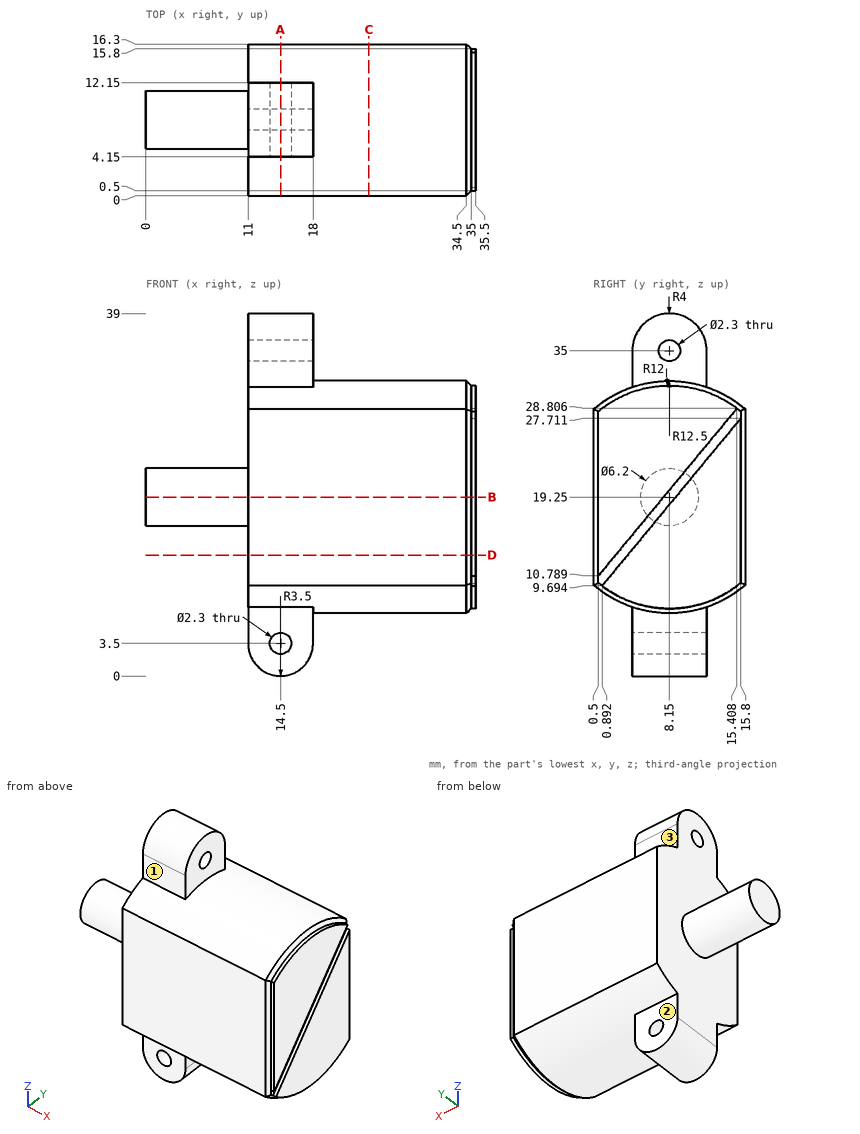
Source: three-view drawing plus pictorial views. Frame: mm from the lowest corner of the part. A direction names the side the tool comes from. Coordinates: 2 decimals unless noted, no trailing zeros. Order: outer loops, then holes, each group sorted by start corner. A loop starts at its lowest first (then second) coordinate and runs counter-clockwise, first axis right, second up.
Item 1: Set-up query: the marked faces 1, 2 and 3. Return all of +Z, -Z, +X, -X, +Y, -Y with unobstructed straight access to the full face (end or side cutting, diameter ignored); none if empty.
Output values:
face 1: +Z, +X, -X, -Y
face 2: -Z, +X, -X, +Y
face 3: +Z, +X, -X, +Y
Item 2: First-contact query: P1, Ø2, axis at y = 8.5, z = 4.5, coming from the +X side; P2, Ø8, axis at x = 27, y = 6.5, coming from the -Z side; P3, Ø2, axis at x = 8.5, z = 15.5, coming from the +Y side. Flat tips, straight axial feed; report the tip coordinate or a pass-through.
Output values:
P1: stops at x = 18
P2: stops at z = 6.75
P3: stops at y = 9.58
Item 3: Material intervals for line 1 (Y direction, x = 15, z = 35); line 2 (X direction, y = 8.5, z = 3.5); line 3 (Z direction, x = 14.5, y = 7.5), sorted ascending.
Output values:
line 1: y = 4.15 to 7, 9.3 to 12.15
line 2: x = 11 to 13.35, 15.65 to 18
line 3: z = 0 to 2.35, 4.65 to 34.05, 35.95 to 38.95
Item 4: Cut plane D-D (z = 13). Return loops of the section in (x, y).
Output values:
outline: (11, 0) - (34.5, 0) - (35, 0.5) - (35.5, 0.5) - (35.5, 2.33) - (35, 2.33) - (35, 3.63) - (35.5, 3.63) - (35.5, 15.8) - (35, 15.8) - (34.5, 16.3) - (11, 16.3) - close
Item 5: Cut plane A-A (x = 14.5). Return loops of the section in (y, z).
Output values:
outline: (0, 9.77) arc R12.5 ccw to (4.15, 7.41) - (4.15, 4.65) - (12.15, 4.65) - (12.15, 7.41) arc R12.5 ccw to (16.3, 9.77) - (16.3, 28.73) arc R12.5 ccw to (12.15, 31.09) - (12.15, 35) arc R4 ccw to (4.15, 35) - (4.15, 31.09) arc R12.5 ccw to (0, 28.73) - close; (4.15, 0) - (12.15, 0) - (12.15, 2.35) - (4.15, 2.35) - close; hole circle Ø2.3 at (8.15, 35)
Item 6: Cut plane C-C (x = 24). Return loops of the section in (y, z), plus the area to 3 significant figures.
Output values:
outline: (0, 9.77) arc R12.5 ccw to (16.3, 9.77) - (16.3, 28.73) arc R12.5 ccw to (0, 28.73) - close
area: 376 mm2
Item 7: Cut plane B-B (z = 19.25). Return loops of the section in (x, y).
Output values:
outline: (0, 5.05) - (11, 5.05) - (11, 0) - (34.5, 0) - (35, 0.5) - (35.5, 0.5) - (35.5, 7.5) - (35, 7.5) - (35, 8.8) - (35.5, 8.8) - (35.5, 15.8) - (35, 15.8) - (34.5, 16.3) - (11, 16.3) - (11, 11.25) - (0, 11.25) - close
